```python
from build123d import *

# Parameters (mm, degrees)
EXTRUDE_1_DEPTH     = 68
SKETCH_2_R          = 2.5
CUT_EXTRUDE_1_DEPTH = 10


with BuildPart() as part:
    # 草图1 → 凸台-拉伸1 (new body)
    with BuildSketch(Plane.XY):
        Polygon((0, 0), (16, 0), (16, -40), (0, -40), (0, -43), (19, -43), (19, 3), (0, 3), align=None)
    extrude(amount=EXTRUDE_1_DEPTH)

    # 草图2 → 切除-拉伸1 (cut)
    with BuildSketch(Plane.XZ.offset(43)):
        with Locations(Location((11, 7.250946933, 0), (0, 0, 270))):
            Circle(SKETCH_2_R)
        with Locations(Location((11, 57.250946933, 0), (0, 0, 270))):
            Circle(SKETCH_2_R)
    extrude(amount=-CUT_EXTRUDE_1_DEPTH, mode=Mode.SUBTRACT)


solid = part.part
```
The model under review builds one solid part; all positions refer to its coordinate system, in mm. A direction names the side the tool comes from. Round coordinates to 2 decimals unless told otherwise and drop trailing zeros. Loops run counter-clockwise (first coordinate to the right, second up) from the corner with the lowest first, then second, coordinate; pieces in that order, holes last. Notation, with made-up numbers: (85, -38.75) - (123, -38.75) arc R22 cw to (123, -16.75) - close; hole circle Ø4 at (64, 3). An arc over 180 degrees is marked (long way). Use a Markdown table: item, result. Add a question column.
Q1. Add section A-A (x = 3.25). State the section outline as (y, z) points.
Q2. Machinability: for faces 5 (the face through (16, -20, 34)), 6 (the face through (9, -43, 34)), 7 (the face through (10.042, -41.521, 54.942)), which of the approach directions +Z, -Z, +X, -X, +Y, -Y give a long, thin tool a straight path to every point of the face, cutting with its end or side? Answer none if there is none.
Q3. Add section B-B (z = 7). State the section outline as (x, y) points.
Q4. For probe 1 along Y at (x, z) = (2.5, 14.5); probe 2 along X at (y, z) = (-6.5, 4), list the stretches that pass through material, from the lowest coordinate up.
Q5. Add section C-C (z = 37). State the section outline as (x, y) points, plus the area to 3 significant figures.
Q6. Add section D-D (x = 11). State the section outline as (y, z) points.
Q7. The part is to be moulded in two halves that separate along X. For faces 1 (the face through (0, -41, 34)), 2 (the face through (9.479, -41.521, 9.235)), 3 (the face through (8, 0, 34)), 4 (the face through (19, -20, 34)), say which applies: pulls with the +X half, pulls with the -X half, needs draft (parallel to the pull), parting line crosses it, or undercut.
Worked answers:
| question | item | result |
|---|---|---|
| 1 | outline | (-43, 0) - (-40, 0) - (-40, 68) - (-43, 68) - close; (0, 0) - (3, 0) - (3, 68) - (0, 68) - close |
| 2 | face 5 | +Z, -Z, -X |
| 2 | face 6 | +Z, -Z, +X, -X, -Y |
| 2 | face 7 | -Y |
| 3 | outline | (0, -43) - (8.51, -43) - (8.51, -40) - (0, -40) - close; (0, 0) - (16, 0) - (16, -40) - (13.49, -40) - (13.49, -43) - (19, -43) - (19, 3) - (0, 3) - close |
| 4 | probe 1 | -43 to -40, 0 to 3 |
| 4 | probe 2 | 16 to 19 |
| 5 | outline | (0, -43) - (19, -43) - (19, 3) - (0, 3) - (0, 0) - (16, 0) - (16, -40) - (0, -40) - close |
| 5 | area | 234 mm² |
| 6 | outline | (-43, 0) - (-40, 0) - (-40, 4.75) - (-43, 4.75) - close; (-43, 9.75) - (-40, 9.75) - (-40, 54.75) - (-43, 54.75) - close; (-43, 59.75) - (-40, 59.75) - (-40, 68) - (-43, 68) - close; (0, 0) - (3, 0) - (3, 68) - (0, 68) - close |
| 7 | face 1 | pulls with the -X half |
| 7 | face 2 | undercut |
| 7 | face 3 | needs draft |
| 7 | face 4 | pulls with the +X half |
